Geometry: final body of the model. Coordinates: model frame, mm. Face numbers are marked on the shaded views. Give positions to 0.01 mm unless a question says otherwise; leave off trailing zeros. Write each loop counter-clockwise with the first axis right and the second up, starting at its lowest first coordinate (ties: lowest second). Pieces come first, ordered by that corner, then holes.
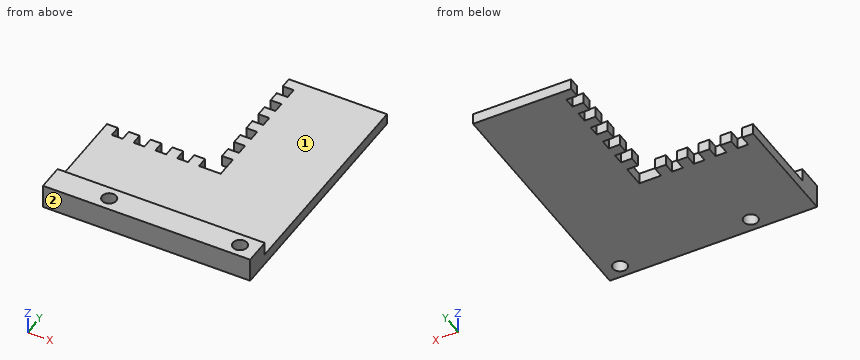
```python
from build123d import *

# Parameters (mm, degrees)
F1_DEPTH = 11
F3_D     = 6.5
F4_D     = 6.5
F5_DEPTH = 5


with BuildPart() as f1:
    # F0 (on Top) → F1 (new body)
    with BuildSketch(Plane.XY):
        Polygon((-19, 0), (0, 0), (76, 0), (76, 12), (0, 12), (-19, 12), align=None)
    extrude(amount=F1_DEPTH)

    # F3 (through all)
    with Locations(Plane.XY.offset(11)):
        with Locations((8, 6)):
            Hole(F3_D / 2)

    # F4 (through all)
    with Locations(Plane.XY.offset(11)):
        with Locations((68, 6)):
            Hole(F4_D / 2)

    # F0 (on Top) → F5 (join)
    with BuildSketch(Plane.XY):
        Polygon((0, 12), (76, 12), (76, 52.551852), (76, 55), (76, 112.551852), (31, 112.551852), (31, 107.551852), (36, 107.551852), (36, 102.551852), (31, 102.551852), (31, 97.551852), (36, 97.551852), (36, 92.551852), (31, 92.551852), (31, 87.551852), (36, 87.551852), (36, 82.551852), (31, 82.551852), (31, 77.551852), (36, 77.551852), (36, 72.551852), (31, 72.551852), (31, 67.551852), (36, 67.551852), (36, 62.551852), (31, 62.551852), (31, 57.551852), (36, 57.551852), (36, 52.551852), (36, 47.551852), (26, 47.551852), (26, 52.551852), (21, 52.551852), (21, 47.551852), (16, 47.551852), (16, 52.551852), (11, 52.551852), (11, 47.551852), (6, 47.551852), (6, 52.551852), (1, 52.551852), (1, 47.551852), (-4, 47.551852), (-4, 52.551852), (-9, 52.551852), (-9, 47.551852), (-14, 47.551852), (-14, 52.551852), (-19, 52.551852), (-19, 47.551852), (-19, 12), align=None)
    extrude(amount=F5_DEPTH)


solid = f1.part
```
Item 1: Section A-A, the plane y = 6. Return the cut outline in (x, z).
Found:
outline: (-19, 0) - (4.75, 0) - (4.75, 11) - (-19, 11) - close; (11.25, 0) - (64.75, 0) - (64.75, 11) - (11.25, 11) - close; (71.25, 0) - (76, 0) - (76, 11) - (71.25, 11) - close
Item 2: Section B-B, the plane x = 8. Return the cut outline in (y, z), plus the area to 3 significant figures.
Found:
outline: (0, 0) - (2.75, 0) - (2.75, 11) - (0, 11) - close; (9.25, 0) - (47.55, 0) - (47.55, 5) - (12, 5) - (12, 11) - (9.25, 11) - close
area: 238 mm2
Item 3: Section C-C, the plane x = 68. Return the cut outline in (y, z), plus the area to 3 significant figures.
Found:
outline: (0, 0) - (2.75, 0) - (2.75, 11) - (0, 11) - close; (9.25, 0) - (112.55, 0) - (112.55, 5) - (12, 5) - (12, 11) - (9.25, 11) - close
area: 563 mm2
Item 4: Pull-direction query (Y, two-part tool) for the marked faces 1 and 2; classes: +Y half, -Y half, draft (parallel to the pull), parting line (faces both ways), or undercut.
Found:
face 1: draft
face 2: -Y half
Item 5: Line query: L1, parallel to Y at x = 8, z = 4.75; L2, parallel to Y at x = 68, z = 3; L3, parallel to X at y = 100.5, z = 3.5. Output: solid intervals per line, ascending.
Found:
L1: y = 0 to 2.75, 9.25 to 47.55
L2: y = 0 to 2.75, 9.25 to 112.55
L3: x = 31 to 76
Item 6: Section D-D, the plane z = 2.5. State how many separate pieces and enclosed holes the cut face has, plus the area to 3 significant figures.
Found:
separate pieces: 1
enclosed holes: 2
area: 7,330 mm2
Item 7: Pin query (flat end, axial travel): pin 1 Ø2.5 at (y, z) = (105, 3.5) entering from -X; pin 2 Ø5 at (x, y) = (55, 23.5) entering from +Z; pin 3 Ø4 at (x, z) = (24, 1.5) entering from +Y. Return the tip coordinate at first contact, or that it passes through.
Found:
pin 1: stops at x = 36
pin 2: stops at z = 5
pin 3: stops at y = 52.55
